Answer from the drawing. Dimensions are ordinates in mm from the lowest x, y and z of the part. Round coordinates to 2 decimals unless told otherwise and drop trailing zeros. Loops run counter-clockwise (first coordinate to the right, second up) from the corner with the lowest first, then second, coordinate; pieces in that order, holes last.
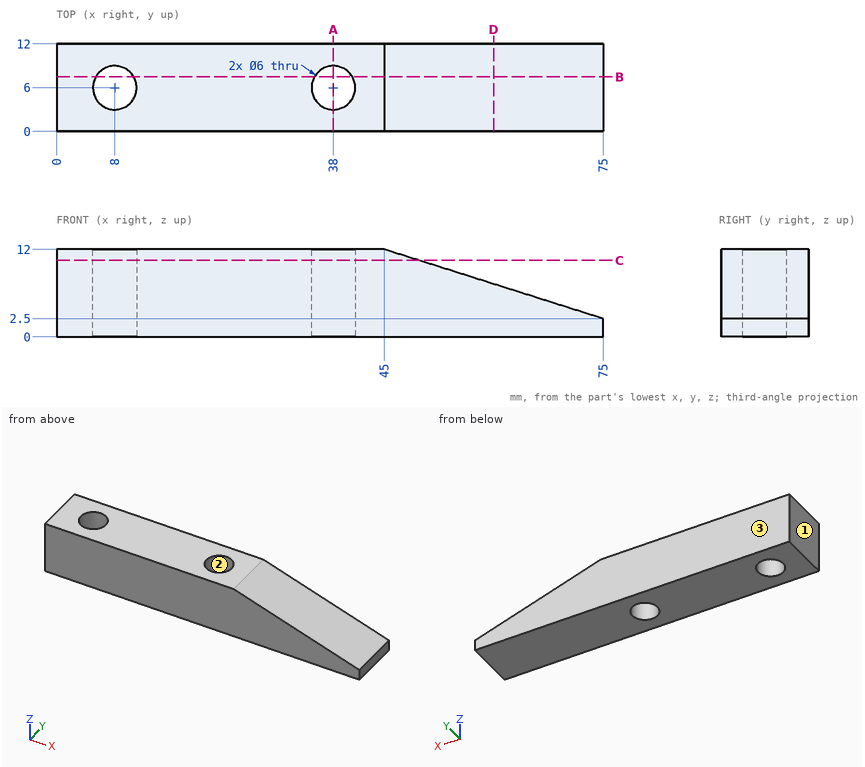
1. Determine the mould class of the marked faces 1, 2 and 3 for opening direction X: +X half, -X half, draft (parallel to the pull), parting line (faces both ways), or undercut.
Answer key:
face 1: -X half
face 2: undercut
face 3: draft
2. Find section D-D (x = 60). Write down the section's boundary in (y, z), then the cut area to 3 significant figures.
Answer key:
outline: (0, 0) - (12, 0) - (12, 7.25) - (0, 7.25) - close
area: 87.0 mm2
3. Find section A-A (x = 38). Write down the section's boundary in (y, z), then the cut area to 3 significant figures.
Answer key:
outline: (0, 0) - (3, 0) - (3, 12) - (0, 12) - close; (9, 0) - (12, 0) - (12, 12) - (9, 12) - close
area: 72.0 mm2
4. Find section B-B (y = 7.5). Write down the section's boundary in (x, z), then the cut area to 3 significant figures.
Answer key:
outline: (0, 0) - (5.4, 0) - (5.4, 12) - (0, 12) - close; (10.6, 0) - (35.4, 0) - (35.4, 12) - (10.6, 12) - close; (40.6, 0) - (75, 0) - (75, 2.5) - (45, 12) - (40.6, 12) - close
area: 633 mm2
5. Find section C-C (z = 10.5). Write down the section's boundary in (x, y).
Answer key:
outline: (0, 0) - (49.74, 0) - (49.74, 12) - (0, 12) - close; hole circle Ø6 at (8, 6); hole circle Ø6 at (38, 6)
6. Consider probe 1 along Y at (x, z) = (8, 5); probe 2 along X at (y, z) = (4.75, 2); probe 3 along Z at (x, y) = (61.5, 4) (3 decimals). Determine where each line is inside the solid, lowest interval first.
Answer key:
probe 1: y = 0 to 3, 9 to 12
probe 2: x = 0 to 5.27, 10.73 to 35.27, 40.73 to 75
probe 3: z = 0 to 6.775
